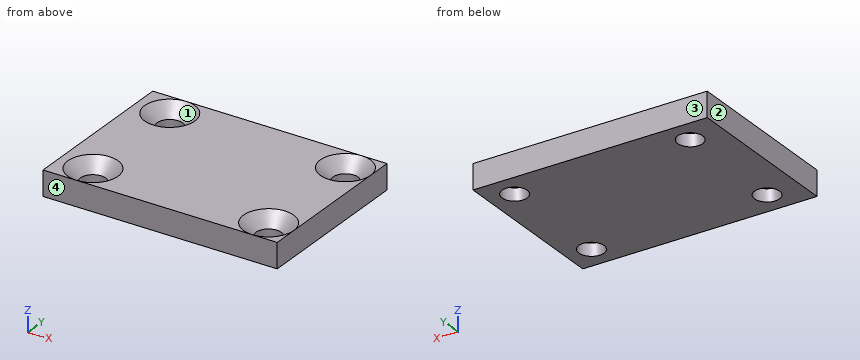
Solid Edge part; units mm, degrees
sketch "Sketch1" plane through (0, 0, 0) normal (0, 0, 1) x (1, 0, 0)
  line L0 (-14, -10) -> (14, -10)
  line L1 (14, -10) -> (14, 10)
  line L2 (14, 10) -> (-14, 10)
  line L3 (-14, 10) -> (-14, -10)
extrude "Protrusion1" add sketch "Sketch1" against normal blind 3
hole "Hole1" at (11, -7, 0) direction (0, 0, -1) diameter 3 end up to next countersink diameter 6 countersink angle 90
hole "Hole2" at (11, 7, 0) direction (0, 0, -1) diameter 3 end up to next countersink diameter 6 countersink angle 90
hole "Hole3" at (-10, 7, 0) direction (0, 0, -1) diameter 3 end up to next countersink diameter 6 countersink angle 90
hole "Hole4" at (-10, -7, 0) direction (0, 0, -1) diameter 3 end up to next countersink diameter 6 countersink angle 90
Can you work these out from the model? Positions are in its coordinate system, mm. Face numbers are marked on the shaded views. Round coordinates to 2 decimals unless told otherwise and drop trailing zeros. Write each loop counter-clockwise with the first axis right and the second up, starting at its lowest first coordinate (ties: lowest second). Pieces come first, ordered by that corner, then holes. Notation, with made-up numbers: (66.25, 4.5) -> (95.25, 4.5) arc R22 cw to (95.25, 20.5) -> close; hole circle Ø6 at (22, -17.5). An arc over 180 degrees is marked (long way). Use one line per item in the form item = value. Start each with the question number.
Q1. If I drill on probe 1 along Y at (x, z) = (-10, -1.95); probe 2 along X at (y, z) = (7, -2.6); probe 3 along X at (y, z) = (-6.75, -1.1), over which ranges is the centre line in solid material (lowest first)? Write a range as [from, to].
Q2. Imagine slicing it at B-B (z = -0.35). Please give me the cut outline in (x, y), then the cut area to 3 significant figures.
Q3. Imagine slicing it at A-A (z = -2.5). Please give me the cut outline in (x, y), then the cut area to 3 significant figures.
Q4. Imagine slicing it at C-C (y = -6.5). Count the separate pieces of the cut face and the enclosed holes in it, then the cut area to 3 significant figures.
Q5. We'd pull the mould along Y, two halves only. Please class the marked faces 1, 2, 3 and 4: +Y half, -Y half, draft (parallel to the pull), parting line (faces both ways), or undercut.
Q6. I'm going to push flat-ended pins straight in: P1, Ø5, axis at x = -10, y = -7, coming from the +Z side; P2, Ø2.5, axis at x = -10, y = 7, coming from the -Z side. Where does each tip first touch, or does it pass through?
Worked out:
q1.probe_1 = [-10, -8.5], [-5.5, 5.5], [8.5, 10]
q1.probe_2 = [-14, -11.5], [-8.5, 9.5], [12.5, 14]
q1.probe_3 = [-14, -11.88], [-8.12, 9.12], [12.88, 14]
q2.outline = (-14, -10) -> (14, -10) -> (14, 10) -> (-14, 10) -> close; hole circle Ø5.3 at (-10, -7); hole circle Ø5.3 at (-10, 7); hole circle Ø5.3 at (11, -7); hole circle Ø5.3 at (11, 7)
q2.area = 472 mm^2
q3.outline = (-14, -10) -> (14, -10) -> (14, 10) -> (-14, 10) -> close; hole circle Ø3 at (-10, -7); hole circle Ø3 at (-10, 7); hole circle Ø3 at (11, -7); hole circle Ø3 at (11, 7)
q3.area = 532 mm^2
q4.separate_pieces = 3
q4.enclosed_holes = 0
q4.area = 62.4 mm^2
q5.face_1 = undercut
q5.face_2 = draft
q5.face_3 = +Y half
q5.face_4 = -Y half
q6.P1 = -0.5
q6.P2 = through
